Check sheet for the drawn part. Datum: minimum x, y, z corner. Units: mm. A direction names the side the tool comes from. Round coordinates to 2 decimals unless told otherwise and drop trailing zeros. Order: outer loops, then holes, each group sorted by start corner. A loop starts at its lowest first (then second) coordinate and runs counter-clockwise, first axis right, second up. Notation, with made-up numbers: (70.25, -18) - (85.25, -18) arc R30 ccw to (85.25, 10) - close; hole circle Ø1 at (62, -8.5). An arc over 180 degrees is marked (long way). Write each question's results on one line, items separated by ' | '.
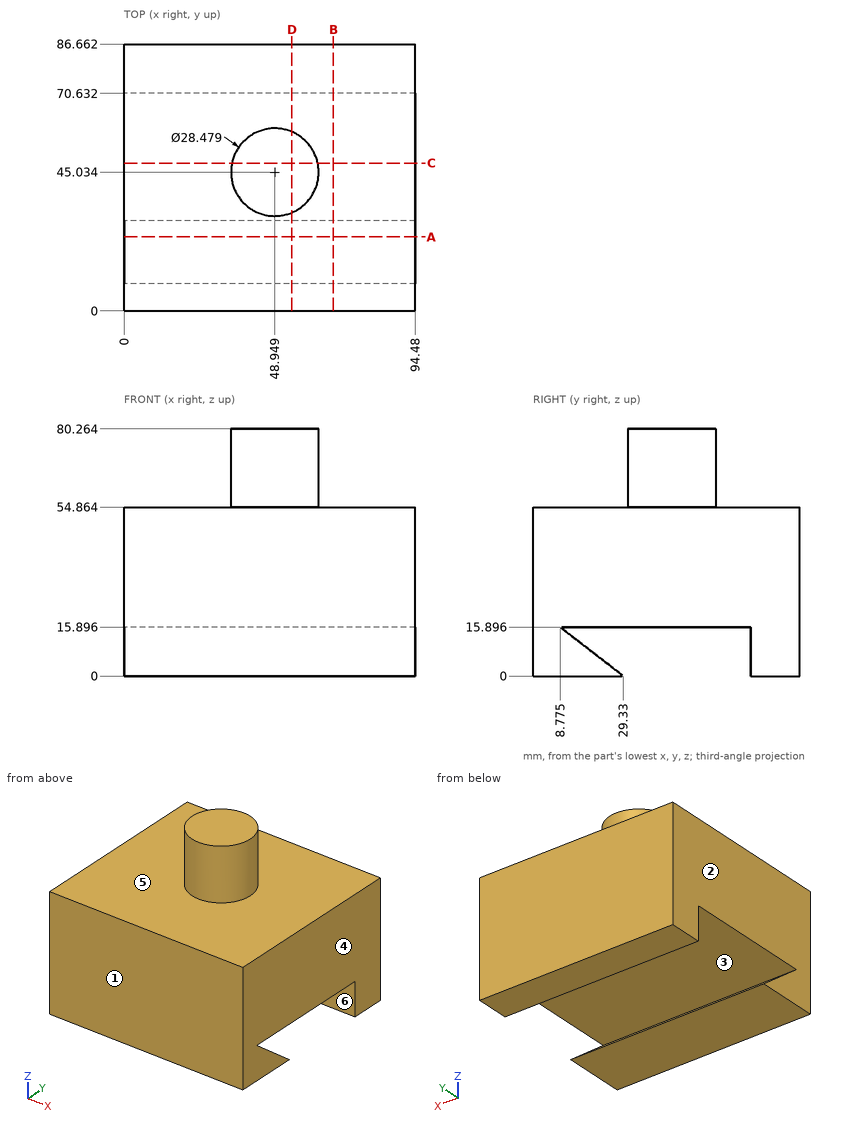
(1) Material ranges on line 1 (Z direction, x = 89, y = 14.5) (1 decimal); line 2 (Z direction, x = 24, y = 68); line 3 (Z direction, x = 36.5, y = 14) (1 decimal), recorded low to high.
Answers follow:
line 1: 0 to 11.5, 15.9 to 54.9 | line 2: 15.9 to 54.86 | line 3: 0 to 11.9, 15.9 to 54.9
(2) Section check D-D (x = 54.5). Record the cut outline in (y, z) (1 decimal), then the cut area to 3 significant figures.
Answers follow:
outline: (0, 0) - (29.3, 0) - (8.8, 15.9) - (70.6, 15.9) - (70.6, 0) - (86.7, 0) - (86.7, 54.9) - (58.1, 54.9) - (58.1, 80.3) - (31.9, 80.3) - (31.9, 54.9) - (0, 54.9) - close | area: 4,600 mm²
(3) Section check B-B (x = 68). Record the cut outline in (y, z) (1 decimal).
Answers follow:
outline: (0, 0) - (29.3, 0) - (8.8, 15.9) - (70.6, 15.9) - (70.6, 0) - (86.7, 0) - (86.7, 54.9) - (0, 54.9) - close
(4) Section check A-A (y = 24). Record the cut outline in (x, z).
Answers follow:
outline: (0, 0) - (94.48, 0) - (94.48, 4.12) - (0, 4.12) - close; (0, 15.9) - (94.48, 15.9) - (94.48, 54.86) - (0, 54.86) - close
(5) Access from +Z, -Z, +X, -X, +Y, -Y to the whole of each face (thin tool, end or side, straight path). Record for the marked faces 4, 5 and 6.
Answers follow:
face 4: +Z, -Z, +X, +Y, -Y | face 5: +Z | face 6: -Z, +X, -X
(6) Depth check by flat-ended pin: pin 1 Ø3 at (x, y) = (49, 53.5) entering from -Z; pin 2 Ø2 at (y, z) = (40, 68.5) entering from +X (1 decimal); pin 3 Ø6 at (x, z) = (44.5, 71) entering from -Y. Enter the tip coordinate at first touch or a pass-through.
Answers follow:
pin 1: z = 15.9 | pin 2: x = 62.6 | pin 3: y = 30.87
(7) Section check C-C (y = 48). Record the cut outline in (x, z).
Answers follow:
outline: (0, 15.9) - (94.48, 15.9) - (94.48, 54.86) - (62.88, 54.86) - (62.88, 80.26) - (35.02, 80.26) - (35.02, 54.86) - (0, 54.86) - close
(8) Draft check along Y on the marked faces 1, 2 and 3. Enter one of: released by +Y, released by -Y, zero draft, split by the parting line, or undercut.
Answers follow:
face 1: released by -Y | face 2: zero draft | face 3: undercut
